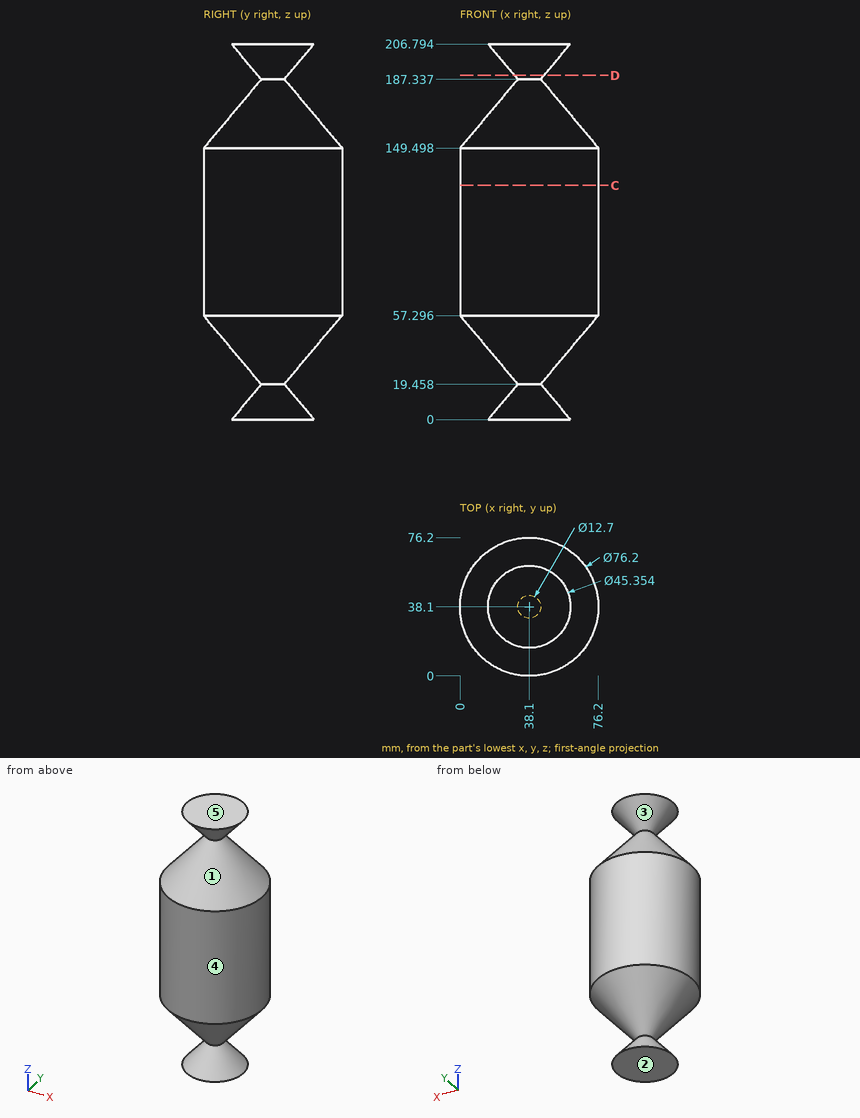
Geometry: see drawing. Coordinates: mm, zero at the bounding-box minimum. A direction names the side the tool comes from. Give positions to 0.01 mm unless a question says otherwise; leave off trailing zeros. Order: outer loops, then holes, each group sorted by start corner. A loop starts at its lowest first (then second) coordinate and runs counter-clockwise, first axis right, second up. Notation, with made-up numbers: M -13.75,35.5 L 30.25,35.5 A20 ccw 30.25,44.5 Z; hole C 65,-37 d6. An arc over 180 degrees is marked long. Answer as CSV lines item,"result". Start each with the question number.
1) First-contact query: P1, Ø4, axis at x = 66, y = 20.5, coming from the +Z side (1 decimal); P2, Ø4, axis at y = 16, z = 153.5, coming from the -X side; P3, Ø6, axis at y = 29.5, z = 155.5, coming from the +X side. Flat tips, straight axial feed; report the tip coordinate or a pass-through.
2) Cut plane C-C (z = 129). Output: boundary loops of the cut face in (x, y).
3) Line query: line 1 (Z direction, x = 57, y = 27) (1 decimal); line 2 (Z direction, x = 26, y = 37.5) (1 decimal); line 3 (X direction, y = 37, z = 123) (1 decimal). Output: solid intervals per line, ascending. Write a range as from..to.
4) Mould query, pull axis Z, two halves, no side actions, for the marked faces 3, 4 and 5. Classes: +Z half, -Z half, draft (parallel to the pull), parting line (faces both ways), or undercut.
5) Cut plane D-D (z = 189.5). Output: boundary loops of the cut face in (x, y) (1 decimal).
6) Set-up query: the marked faces 1 and 2. Return all of +Z, -Z, +X, -X, +Y, -Y with unobstructed straight access to the full face (end or side cutting, diameter ignored); none if empty.
Findings below:
1,P1,"stops at z = 158"
1,P2,"stops at x = 8.68"
1,P3,"stops at x = 72.72"
2,outline,"C 38.1,38.1 d76.2"
3,line 1,"z = 0..0.9, 38..168.8, 205.9..206.8"
3,line 2,"z = 0..12.6, 26.3..180.5, 194.2..206.8"
3,line 3,"x = 0..76.2"
4,face 3,"undercut"
4,face 4,"draft"
4,face 5,"+Z half"
5,outline,"C 38.1,38.1 d16.3"
6,face 1,"none"
6,face 2,"-Z, +X, -X, +Y, -Y"
